```python
from build123d import *

# Parameters (mm, degrees)
RESSALTO_EXTRUS_O1_DEPTH   = 15
CORTE_EXTRUS_O1_DEPTH      = 26.475478406
CORTE_EXTRUS_O1_DEPTH_BACK = 26.475478406
ESBO_O2_R                  = 1.45


with BuildPart() as part:
    # Esboço1 → Ressalto-extrusão1 (new body)
    with BuildSketch(Plane.XY):
        Polygon((0, 0), (17.8325545, 10.295630141), (17.8325545, 0.295630141), (17.8325545, -2), (0, -2), align=None)
    extrude(amount=RESSALTO_EXTRUS_O1_DEPTH)

    # Esboço2 → Corte-extrusão1 (cut, two sides: drawn at the far end of the back side and taken through both)
    with BuildSketch(Plane.XY.offset(15).offset(-CORTE_EXTRUS_O1_DEPTH_BACK)):
        with Locations((14.8325545, 3)):
            Circle(ESBO_O2_R)
    extrude(amount=CORTE_EXTRUS_O1_DEPTH + CORTE_EXTRUS_O1_DEPTH_BACK, mode=Mode.SUBTRACT)


solid = part.part
```
Check sheet for the modelled part. Datum: model origin and axes. Units: mm. Give positions to 0.01 mm unless a question says otherwise; leave off trailing zeros. Write each loop counter-clockwise with the first axis right and the second up, starting at its lowest first coordinate (ties: lowest second). Pieces come first, ordered by that corner, then holes. Notation, with made-up numbers: (44, -35) -> (57, -35) arc R14 ccw to (57, -11) -> close; hole circle Ø7 at (76.25, 28.5). An arc over 180 degrees is marked (long way). Use CSV: the item, a comma, the result in double quotes. Start each with the question number.
Q1. Release check for a two-part mould opening along X. For faces 1 (the flat face through (9, -2, 7)), 2 (the flat face through (17.833, 4, 7)), 3 (the cylindrical face through (13.384, 3.064, 7.395)) record: +X half, -X half, draft (parallel to the pull), parting line (faces both ways), or undercut.
Q2. Depth check by flat-ended pin: P1, Ø3, axis at x = 13.5, y = 3.5, coming from the +Z side; P2, Ø2.5, axis at x = 14.83, y = 3, coming from the -Z side; P3, Ø1.5, axis at x = 4.5, z = 1.5, coming from the +Y side; P4, Ø4, axis at x = 2.5, z = 7.5, coming from the +Y side. Enter the tip coordinate at first touch or a pass-through.
Q3. Cross-section at B-B on z = 7. Enter the section's corners in (x, y), and give its area (3 significant figures).
Q4. Cross-section at A-A on y = 3. Enter the section's corners in (x, z), and give its area (3 significant figures).
Q5. Cross-section at D-D on y = 6. Enter the section's corners in (x, z), and give its area (3 significant figures).
Q6. Scan lines: line 1 along X through (y, z) = (3, 10.75); line 2 along X through (y, z) = (2.5, 11.75); line 3 along Y through (x, z) = (12.5, 12). Record each from-to range of solid material in increasing order.
Q7. Cross-section at C-C on x = 8.75. Enter the section's corners in (y, z).
Working result:
1,face 1,"draft"
1,face 2,"+X half"
1,face 3,"undercut"
2,P1,"stops at z = 15"
2,P2,"passes through"
2,P3,"stops at y = 3.03"
2,P4,"stops at y = 2.6"
3,outline,"(0, -2) -> (17.83, -2) -> (17.83, 10.3) -> (0, 0) -> close; hole circle Ø2.9 at (14.83, 3)"
3,area,"121 mm^2"
4,outline,"(5.2, 0) -> (13.38, 0) -> (13.38, 15) -> (5.2, 15) -> close; (16.28, 0) -> (17.83, 0) -> (17.83, 15) -> (16.28, 15) -> close"
4,area,"146 mm^2"
5,outline,"(10.39, 0) -> (17.83, 0) -> (17.83, 15) -> (10.39, 15) -> close"
5,area,"112 mm^2"
6,line 1,"x = 5.2 to 13.38, 16.28 to 17.83"
6,line 2,"x = 4.33 to 13.47, 16.19 to 17.83"
6,line 3,"y = -2 to 7.22"
7,outline,"(-2, 0) -> (5.05, 0) -> (5.05, 15) -> (-2, 15) -> close"
